Autodesk Inventor part; units mm, degrees
ref_plane "YZ Plane" through (0, 0, 0) normal (1, 0, 0) x (0, 1, 0)
ref_plane "XZ Plane" through (0, 0, 0) normal (0, 1, 0) x (-1, 0, 0)
ref_plane "XY Plane" through (0, 0, 0) normal (0, 0, 1) x (1, 0, 0)
sketch "スケッチ1" plane through (0, 0, 0) normal (0, 0, 1) x (1, 0, 0)
  circle A0 centre (0, 0) radius 10
  line L0 (-11.3487, 8.25) -> (5.6513, 8.25)
  line L1 (5.6513, 8.25) -> (5.6513, -8.25)
  line L2 (5.6513, -8.25) -> (-11.3487, -8.25)
  line L3 (-11.3487, -8.25) -> (-11.3487, 8.25)
  point P0 (5.6513, 0)
  point P1 (-5.6513, 8.25)
  point P2 (-5.6513, -8.25)
  dimension "d0" = 20
  dimension "d1" = 16.5
  dimension "d2" = 17
extrude "押し出し1" add sketch "スケッチ1" along normal blind 2 contours L0 A0 | L1 L2 A0 L0 | A0 L2 | A0 L2 L3 L0
sketch "スケッチ2" plane through (0, 0, 2) normal (0, 0, 1) x (1, 0, 0)
  circle A0 centre (0, 0) radius 2.5
  dimension "d5" = 5
extrude "押し出し2" cut sketch "スケッチ2" against normal blind 2
properties part number "encoder"
For this review, take the finished solid that the model builds, in its own axes (mm). A direction names the side the tool comes from. Give positions to 0.01 mm unless a question says otherwise; leave off trailing zeros. Order: outer loops, then holes, each group sorted by start corner. A loop starts at its lowest first (then second) coordinate and runs counter-clockwise, first axis right, second up. Notation, with made-up numbers: (-25, -33.75) -> (5, -33.75) arc R11 ccw to (5, -20.75) -> close; hole circle Ø5 at (38, 50.25). An arc over 180 degrees is marked (long way). Write item = value, one per line.
1) We need section D-D, the plane x = -8.25. Give the boundary of the cut face in (y, z), and give its area (3 significant figures).
Findings:
outline = (-8.25, 0) -> (8.25, 0) -> (8.25, 2) -> (-8.25, 2) -> close
area = 33.0 mm^2
2) To check wall thickness, follow L1, parallel to Y at x = 0, z = 0.6; L2, parallel to Y at x = -8.5, z = 1.75; L3, parallel to X at y = 1, z = 0.15. State the ranges of each line that lie inside material, in increasing order. Write a range as from..to.
Findings:
L1 = -10..-2.5, 2.5..10
L2 = -8.25..8.25
L3 = -11.35..-2.29, 2.29..5.65
3) For faces 1 (the face through (-8, -8.25, 1)), 2 (the face through (0, -10, 1)), 3 (the face through (-9, 8.25, 1)), list the 3-axis set-ups (+Z, -Z, +X, -X, +Y, -Y) from which the entire face can be reached by the end or side of a thin tool; tool diameter is ignored.
Findings:
face_1 = +Z, -Z, -X, -Y
face_2 = +Z, -Z, -Y
face_3 = +Z, -Z, -X, +Y
4) We need section C-C, the plane z = 0.6. Give the boundary of the cut face in (x, y), and give its area (3 significant figures).
Findings:
outline = (-11.35, -8.25) -> (-5.65, -8.25) arc R10 ccw to (5.65, -8.25) -> (5.65, 8.25) arc R10 ccw to (-5.65, 8.25) -> (-11.35, 8.25) -> close; hole circle Ø5 at (0, 0)
area = 288 mm^2
5) We need section B-B, the plane x = 0. Give the boundary of the cut face in (y, z).
Findings:
outline = (-10, 0) -> (-2.5, 0) -> (-2.5, 2) -> (-10, 2) -> close; (2.5, 0) -> (10, 0) -> (10, 2) -> (2.5, 2) -> close
6) Draft analysis for pull direction X (two halves, no side actions). For faces 4 (the face through (5.651, 0, 1)), 5 (the face through (0, 10, 1)), 6 (the face through (-0.54, -2.44, 1.01)), state which applies: pulls with the +X half, pulls with the -X half, needs draft (parallel to the pull), parting line crosses it, or undercut.
Findings:
face_4 = pulls with the +X half
face_5 = parting line crosses it
face_6 = undercut
7) We need section A-A, the plane y = 0. Give the boundary of the cut face in (x, z), and give its area (3 significant figures).
Findings:
outline = (-11.35, 0) -> (-2.5, 0) -> (-2.5, 2) -> (-11.35, 2) -> close; (2.5, 0) -> (5.65, 0) -> (5.65, 2) -> (2.5, 2) -> close
area = 24.0 mm^2
8) Insertion check: pin 1 (1 mm diameter, centred on x = -8, z = 0.5, fed in from +Y); pin 2 (1 mm diameter, centred on x = -8.5, z = 1, fed in from -Y). Each pin has a flat end and moves straight along its axis. Give the tip position at first contact, or say it passes through.
Findings:
pin_1 = 8.25
pin_2 = -8.25
